Read the model definition and answer for the solid it produces. Units are mm, in the model's axes. Face numbers are marked on the shaded views. A direction names the side the tool comes from. Give positions to 0.01 mm unless a question says otherwise; leave off trailing zeros. Write each loop counter-clockwise with the first axis right and the second up, starting at its lowest first coordinate (ties: lowest second). Pieces come first, ordered by that corner, then holes. Notation, with made-up numbers: M -26.75,86 L 19.25,86 A23 ccw 19.25,95 Z; hole C -10.75,-25 d6. An arc over 180 degrees is marked long. Answer as CSV lines item,"result". Start each with the question number.
```python
from build123d import *

# Parameters (mm, degrees)
BOSS_EXTRUDE1_DEPTH = 13
BOSS_EXTRUDE7_DEPTH = 9
SKETCH2_R           = 12
CUT_EXTRUDE1_DEPTH  = 4.5
CUT_EXTRUDE3_DEPTH  = 6.5
SKETCH6_R           = 1.57
CUT_EXTRUDE4_DEPTH  = 13
BOSS_EXTRUDE2_DEPTH = 0.85
BOSS_EXTRUDE3_START = 0.85
BOSS_EXTRUDE3_DEPTH = 0.85
SKETCH3_R           = 4.12
BEARING_AXIS_DEPTH  = 10
CHAMFER1_SIZE       = 0.85
CUT_EXTRUDE6_DEPTH  = 2
CUT_EXTRUDE7_DEPTH  = 2
SKETCH15_W          = 20
SKETCH15_H          = 4
BOSS_EXTRUDE4_DEPTH = 6
FILLET1_R           = 3.5
FILLET2_R           = 3
FILLET3_R           = 1
SKETCH16_R          = 1
BOSS_EXTRUDE5_DEPTH = 9
FILLET4_R           = 0.6
CUT_EXTRUDE8_DEPTH  = 12
FILLET5_R           = 0.6
FILLET6_R           = 0.5


with BuildPart() as part:
    # Sketch1 → Boss-Extrude1 (new, symmetric)
    with BuildSketch(Plane(origin=(0, 0, 0), x_dir=(0, 0, -1), z_dir=(1, 0, 0))):
        with BuildLine():
            Line((10, -0.346), (2.551698211, -4.645302599))
            ThreePointArc((2.551698211, -4.645302599), (-4.784687849, -2.279640803), (-2, 4.908156477))
            Line((-2, 4.908156477), (-2, 37.654))
            Line((-2, 37.654), (10, 37.654))
            Line((10, 37.654), (10, -0.346))
        make_face()
    extrude(amount=BOSS_EXTRUDE1_DEPTH, both=True)

    # Sketch17 → Boss-Extrude7 (add)
    with BuildSketch(Plane(origin=(0, 37.654, 0), x_dir=(1, 0, 0), z_dir=(0, 1, 0))):
        with BuildLine():
            Line((-4, -2), (4, -2))
            Line((4, -2), (4, -13.8))
            Line((4, -13.8), (1.175, -13.8))
            Line((1.175, -13.8), (1.175, -10.8))
            ThreePointArc((1.175, -10.8), (0, -9.625), (-1.175, -10.8))
            Line((-1.175, -10.8), (-1.175, -13.8))
            Line((-1.175, -13.8), (-4, -13.8))
            Line((-4, -13.8), (-4, -2))
        make_face()
    extrude(amount=-BOSS_EXTRUDE7_DEPTH)

    # Sketch2 → Cut-Extrude1 (cut, symmetric)
    with BuildSketch(Plane(origin=(0, 0, 0), x_dir=(0, 0, -1), z_dir=(1, 0, 0))):
        with Locations((0, 17)):
            Circle(SKETCH2_R)
    extrude(amount=CUT_EXTRUDE1_DEPTH, both=True, mode=Mode.SUBTRACT)

    # Sketch4 → Cut-Extrude3 (cut, symmetric)
    with BuildSketch(Plane(origin=(0, 0, 0), x_dir=(0, 0, -1), z_dir=(1, 0, 0))):
        with BuildLine():
            Line((5.196447381, 2.99948906), (7.845401268, -1.589675699))
            Line((7.845401268, -1.589675699), (7.845401268, -2.399293943))
            Line((7.845401268, -2.399293943), (2.99948906, -5.196447381))
            ThreePointArc((2.99948906, -5.196447381), (-5.795402235, 1.553484127), (5.196447381, 2.99948906))
        make_face()
    extrude(amount=CUT_EXTRUDE3_DEPTH, both=True, mode=Mode.SUBTRACT)

    # Sketch6 → Cut-Extrude4 (cut, symmetric)
    with BuildSketch(Plane(origin=(0, 0, 0), x_dir=(0, 0, -1), z_dir=(1, 0, 0))):
        Circle(SKETCH6_R)
    extrude(amount=CUT_EXTRUDE4_DEPTH, both=True, mode=Mode.SUBTRACT)

    # Sketch8 → Boss-Extrude2 (add)
    with BuildSketch(Plane(origin=(-4.5, 0, 0), x_dir=(0, 0, -1), z_dir=(1, 0, 0))):
        with BuildLine():
            Line((-2, 23.499230724), (-2, 10.500769276))
            ThreePointArc((-2, 10.500769276), (6.8, 17), (-2, 23.499230724))
        make_face()
    extrude(amount=BOSS_EXTRUDE2_DEPTH)

    # Sketch9 → Boss-Extrude3 (add)
    with BuildSketch(Plane.ZY.offset(-4.5).offset(BOSS_EXTRUDE3_START)):
        with BuildLine():
            Line((2, 23.499230724), (2, 10.500769276))
            ThreePointArc((2, 10.500769276), (-6.8, 17), (2, 23.499230724))
        make_face()
    extrude(amount=-BOSS_EXTRUDE3_DEPTH)

    # Sketch3 → bearing_axis (cut, symmetric)
    with BuildSketch(Plane(origin=(0, 0, 0), x_dir=(0, 0, -1), z_dir=(1, 0, 0))):
        with Locations((0, 17)):
            Circle(SKETCH3_R)
    extrude(amount=BEARING_AXIS_DEPTH, both=True, mode=Mode.SUBTRACT)

    # Chamfer1
    chamfer1_edges = [part.edges().sort_by_distance(p)[0] for p in [
        (3.65, 17, -6.8),
        (-3.65, 17, -6.8),
    ]]
    chamfer(chamfer1_edges, length=CHAMFER1_SIZE - 0.0001)  # a hair under: the kernel refuses the full size

    # Sketch12 → Cut-Extrude6 (cut)
    with BuildSketch(Plane(origin=(-6.5, 0, 0), x_dir=(0, 0, -1), z_dir=(1, 0, 0))):
        Polygon((2.650037736, 0), (1.325018868, 2.295), (-1.325018868, 2.295), (-2.650037736, 0), (-1.325018868, -2.295), (1.325018868, -2.295), align=None)
    extrude(amount=-CUT_EXTRUDE6_DEPTH, mode=Mode.SUBTRACT)

    # Sketch14 → Cut-Extrude7 (cut)
    with BuildSketch(Plane.ZY.offset(-6.5)):
        Polygon((-2.650037736, 0), (-1.325018868, -2.295), (1.325018868, -2.295), (2.650037736, 0), (1.325018868, 2.295), (-1.325018868, 2.295), align=None)
    extrude(amount=-CUT_EXTRUDE7_DEPTH, mode=Mode.SUBTRACT)

    # Sketch15 → Boss-Extrude4 (add)
    with BuildSketch(Plane(origin=(0, 37.654, 0), x_dir=(1, 0, 0), z_dir=(0, 1, 0))):
        with Locations((0, 8)):
            Rectangle(SKETCH15_W, SKETCH15_H)
    extrude(amount=BOSS_EXTRUDE4_DEPTH)

    # Fillet1
    fillet1_edges = [part.edges().sort_by_distance(p)[0] for p in [
        (0, 37.654, -6),
    ]]
    fillet(fillet1_edges, radius=FILLET1_R)

    # Fillet2
    fillet2_edges = [part.edges().sort_by_distance(p)[0] for p in [
        (-13, 37.654, -4),
        (13, 37.654, -4),
    ]]
    fillet(fillet2_edges, radius=FILLET2_R - 0.0001)  # a hair under: the kernel refuses the full size

    # Fillet3
    fillet3_edges = [part.edges().sort_by_distance(p)[0] for p in [
        (-10, 43.654, -8),
        (10, 43.654, -8),
    ]]
    fillet(fillet3_edges, radius=FILLET3_R)

    # Sketch16 → Boss-Extrude5 (add, symmetric)
    with BuildSketch(Plane(origin=(0, 0, 0), x_dir=(0, 0, -1), z_dir=(1, 0, 0))):
        with Locations((6, 42.654)):
            Circle(SKETCH16_R)
    extrude(amount=BOSS_EXTRUDE5_DEPTH, both=True)

    # Fillet4
    fillet4_edges = [part.edges().sort_by_distance(p)[0] for p in [
        (-9, 42.654, -5),
        (9, 42.654, -5),
    ]]
    fillet(fillet4_edges, radius=FILLET4_R)

    # Sketch18 → Cut-Extrude8 (cut)
    with BuildSketch(Plane.XY.offset(-10)):
        with BuildLine():
            Line((-10.1, 30.654), (-10.1, 32.654))
            ThreePointArc((-10.1, 32.654), (-8, 34.754), (-5.9, 32.654))
            Line((-5.9, 32.654), (-5.9, 30.654))
            ThreePointArc((-5.9, 30.654), (-8, 28.554), (-10.1, 30.654))
        make_face()
        with BuildLine():
            Line((10.1, 32.654), (10.1, 30.654))
            ThreePointArc((10.1, 30.654), (8, 28.554), (5.9, 30.654))
            Line((5.9, 30.654), (5.9, 32.654))
            ThreePointArc((5.9, 32.654), (8, 34.754), (10.1, 32.654))
        make_face()
    extrude(amount=CUT_EXTRUDE8_DEPTH, mode=Mode.SUBTRACT)

    # Fillet5
    fillet5_edges = [part.edges().sort_by_distance(p)[0] for p in [
        (2.5875, 28.654, 13.8),
        (4, 33.154, 13.8),
        (1.175, 28.654, 12.3),
        (1.175, 33.154, 13.8),
        (0, 28.654, 9.625),
        (-1.175, 28.654, 12.3),
        (-2.5875, 28.654, 13.8),
        (-1.175, 33.154, 13.8),
        (-4, 33.154, 13.8),
        (2.5875, 37.654, 13.8),
        (-2.5875, 37.654, 13.8),
        (-1.175, 37.654, 12.3),
        (0, 37.654, 9.625),
        (1.175, 37.654, 12.3),
    ]]
    fillet(fillet5_edges, radius=FILLET5_R)

    # Fillet6
    fillet6_edges = [part.edges().sort_by_distance(p)[0] for p in [
        (-10.1, 31.654, 2),
        (-8, 34.754, 2),
        (-5.9, 31.654, 2),
        (-8, 28.554, 2),
        (10.1, 31.654, 2),
        (8, 28.554, 2),
        (5.9, 31.654, 2),
        (8, 34.754, 2),
    ]]
    fillet(fillet6_edges, radius=FILLET6_R)


solid = part.part
```
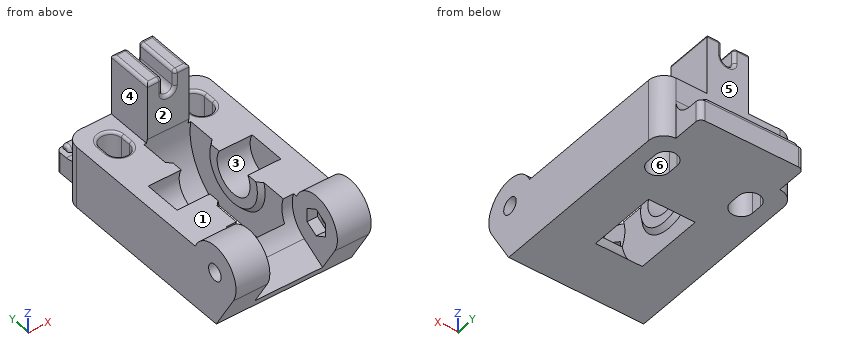
1. Find the intervals of material crossed by line 1 (Y direction, x = 8, z = 0) (3 decimals); line 2 (X direction, y = 37, z = 10.75); line 3 (X direction, y = 21, z = 0.25), in increasing order. Write a range as [from, to].
2. Determine the mould class of the marked faces 1, 2 and 3 for opening direction Z: +Z half, -Z half, draft (parallel to the pull), parting line (faces both ways), or undercut.
3. Find section C-C on z = 0. State how many separate pieces and enclosed holes the cut face has, then the cut area to 3 significant figures.
4. Given pin 1 (1 mm diameter, centred on x = 7, z = 0.5, fed in from +Y); pin 2 (2.5 mm diameter, centred on y = 34, z = 7.5, fed in from +X); pin 3 (2 mm diameter, centred on x = 9, z = 3.5, fed in from -Y); pin 4 (1.5 mm diameter, centred on x = -6, z = 6.5, fed in from +Y), each flat-ended and moving along its own axis, determine where each tip first touches the part or whether it passes through.
5. Find section A-A on y = 32. Determine the outline of the cut face in (x, z) (3 decimals), then the cut area to 3 significant figures.
6. Find section B-B on x = 0. Determine the outline of the cut face in (y, z) (3 decimals), then the cut area to 3 significant figures.
7. For the marked faces 4, 5 and 6, determine the directions among +Z, -Z, +X, -X, +Y, -Y from which every point of the face is accessible in a straight line to the end or side of a thin tool.
Computed:
1,line 1,"y = [-5.3, -2.295], [2.295, 12.88], [21.12, 28.554], [34.754, 37.654]"
1,line 2,"x = [-4, -1.17], [1.17, 4]"
1,line 3,"x = [-13, -10], [10, 13]"
2,face 1,"+Z half"
2,face 2,"draft"
2,face 3,"undercut"
3,separate pieces,"3"
3,enclosed holes,"2"
3,area,"585 mm^2"
4,pin 1,"stops at y = 37.65"
4,pin 2,"stops at x = 4"
4,pin 3,"stops at y = -4.67"
4,pin 4,"passes through"
5,outline,"M -13,-10 L -10.1,-10 L -10.1,1.5 A0.5 ccw -10.6,2 L -13,2 Z; M -5.9,-10 L 5.9,-10 L 5.9,1.5 A0.5 ccw 5.4,2 L 4,2 L 4,13.2 A0.6 ccw 3.4,13.8 L 1.775,13.8 A0.6 ccw 1.175,13.2 L 1.175,10.8 A1.175 cw -1.175,10.8 L -1.175,13.2 A0.6 ccw -1.775,13.8 L -3.4,13.8 A0.6 ccw -4,13.2 L -4,2 L -5.4,2 A0.5 ccw -5.9,1.5 Z; M 10.1,-10 L 13,-10 L 13,2 L 10.6,2 A0.5 ccw 10.1,1.5 Z"
5,area,"296 mm^2"
6,outline,"M -1.59,-7.845 L -0.346,-10 L 10.367,-10 A12 cw 5.324,-2.768 A6 cw 2.999,-5.196 Z; M 23.633,-10 L 43.654,-10 L 43.654,-6 A1 ccw 41.654,-6 L 41.154,-6 A3.5 cw 37.654,-2.5 L 37.654,9.025 A0.6 ccw 37.054,9.625 L 29.254,9.625 A0.6 ccw 28.654,9.025 L 28.654,2.861 A12 cw Z"
6,area,"258 mm^2"
7,face 4,"+Z, -X, +Y, -Y"
7,face 5,"+Z, +X, -X, +Y"
7,face 6,"+Z, -Z"
